from build123d import *

# Parameters (mm, degrees)
SKETCH_1_W          = 45
SKETCH_1_H          = 40
EXTRUDE_1_DEPTH     = 2
EXTRUDE_2_DEPTH     = 20
SKETCH_3_W          = 31
SKETCH_3_H          = 63
EXTRUDE_3_DEPTH     = 2
SKETCH_4_R          = 1.65
CUT_EXTRUDE_1_DEPTH = 2
FILLET_2_R          = 2
EXTRUDE_4_DEPTH     = 20
CUT_EXTRUDE_2_DEPTH = 2.5
CUT_EXTRUDE_5_REACH = 62.26
SKETCH_11_W         = 2
SKETCH_11_H         = 20
FILLET_5_R          = 1
CUT_EXTRUDE_6_DEPTH = 2.5


with BuildPart() as part:
    # 草图1 → 凸台-拉伸1 (new body)
    with BuildSketch(Plane(origin=(0, 0, 0), x_dir=(1, 0, 0), z_dir=(0, 1, 0))):
        Rectangle(SKETCH_1_W, SKETCH_1_H)
    extrude(amount=EXTRUDE_1_DEPTH)

    # 草图2 → 凸台-拉伸2 (add)
    with BuildSketch(Plane(origin=(0, 2, 0), x_dir=(1, 0, 0), z_dir=(0, 1, 0))):
        Polygon((21.5, -2.3), (22.5, -2.3), (22.5, 20), (-22.5, 20), (-22.5, -2.3), (-21.5, -2.3), (-21.5, 19), (21.5, 19), align=None)
    extrude(amount=EXTRUDE_2_DEPTH)

    # 草图3 → 凸台-拉伸3 (add)
    with BuildSketch(Plane.XZ):
        with Locations((0, 2)):
            Rectangle(SKETCH_3_W, SKETCH_3_H)
    extrude(amount=-EXTRUDE_3_DEPTH)

    # 草图4 → 切除-拉伸1 (cut)
    with BuildSketch(Plane.XZ):
        with Locations(Location((0, -23.15, 0), (0, 0, 270))):
            Circle(SKETCH_4_R)
        with Locations(Location((0, 24.35, 0), (0, 0, 90))):
            Circle(SKETCH_4_R)
    extrude(amount=-CUT_EXTRUDE_1_DEPTH, mode=Mode.SUBTRACT)

    # 圆角2
    fillet_2_edges = [part.edges().sort_by_distance(p)[0] for p in [
        (-15.5, 1, -29.5),
        (15.5, 1, 33.5),
        (-15.5, 1, 33.5),
        (15.5, 1, -29.5),
        (22.5, 1, 20),
        (-22.5, 1, 20),
        (-22.5, 11, -20),
        (22.5, 11, -20),
    ]]
    fillet(fillet_2_edges, radius=FILLET_2_R)

    # 草图7 → 凸台-拉伸4 (add)
    with BuildSketch(Plane(origin=(0, 2, 0), x_dir=(1, 0, 0), z_dir=(0, 1, 0))):
        Polygon((20.5, 18), (20.5, -2.3), (21.5, -2.3), (21.5, 19), (20.5, 19), align=None)
        Polygon((-21.5, 19), (-21.5, -2.3), (-20.5, -2.3), (-20.5, 18), (-20.5, 19), align=None)
    extrude(amount=EXTRUDE_4_DEPTH)

    # 草图8 → 切除-拉伸2 (cut)
    with BuildSketch(Plane(origin=(20, 1.9, 0.9), x_dir=(0, 1, 0), z_dir=(1, 0, 0))):
        with BuildLine():
            ThreePointArc((18.33276934, -17.5), (17.54276934, -16.71), (16.75276934, -17.5))
            ThreePointArc((16.75276934, -17.5), (17.54276934, -18.29), (18.33276934, -17.5))
        make_face()
        with BuildLine():
            ThreePointArc((3.33276934, -17.5), (2.54276934, -16.71), (1.75276934, -17.5))
            ThreePointArc((1.75276934, -17.5), (2.54276934, -18.29), (3.33276934, -17.5))
        make_face()
        with BuildLine():
            ThreePointArc((3.33276934, -2.5), (2.54276934, -1.71), (1.75276934, -2.5))
            ThreePointArc((1.75276934, -2.5), (2.54276934, -3.29), (3.33276934, -2.5))
        make_face()
        with BuildLine():
            ThreePointArc((18.33276934, -2.5), (17.54276934, -1.71), (16.75276934, -2.5))
            ThreePointArc((16.75276934, -2.5), (17.54276934, -3.29), (18.33276934, -2.5))
        make_face()
    extrude(amount=CUT_EXTRUDE_2_DEPTH, mode=Mode.SUBTRACT)

    # 切除-拉伸5: up to this face of the body (flat: up to its plane)
    cut_extrude_5_end = Plane(part.part.faces().sort_by_distance((22.5, 10.316412164, -6.626998027))[0])
    # 草图11 → 切除-拉伸5 (cut, up to the picked face)
    with BuildSketch(Plane.ZY.offset(22.5), mode=Mode.PRIVATE) as cut_extrude_5_sk1:
        with Locations((1.3, 12)):
            Rectangle(SKETCH_11_W, SKETCH_11_H)
    cut_extrude_5_tool1 = split(extrude(cut_extrude_5_sk1.sketch, amount=-CUT_EXTRUDE_5_REACH, mode=Mode.PRIVATE), bisect_by=cut_extrude_5_end, keep=Keep.BOTH, mode=Mode.PRIVATE)
    add(cut_extrude_5_tool1.solids().sort_by(Axis((-22.5, 12, 1.3), (1, 0, 0)))[0], mode=Mode.SUBTRACT)

    # 圆角5
    fillet_5_edges = [part.edges().sort_by_distance(p)[0] for p in [
        (20.5, 12, -19),
        (-20.5, 12, -19),
    ]]
    fillet(fillet_5_edges, radius=FILLET_5_R)

    # 草图12 → 切除-拉伸6 (cut)
    with BuildSketch(Plane(origin=(-20, 1.9, 0.9), x_dir=(0, -1, 0), z_dir=(-1, 0, 0))):
        with BuildLine():
            Line((-10.8, -17.95), (-10.8, -16.45))
            ThreePointArc((-10.8, -16.45), (-10, -15.65), (-9.2, -16.45))
            Line((-9.2, -16.45), (-9.2, -17.95))
            ThreePointArc((-9.2, -17.95), (-10, -18.75), (-10.8, -17.95))
        make_face()
        with BuildLine():
            Line((-3.8, -11.0010906), (-3.8, -10.0010906))
            ThreePointArc((-3.8, -10.0010906), (-3, -9.2010906), (-2.2, -10.0010906))
            Line((-2.2, -10.0010906), (-2.2, -11.0010906))
            ThreePointArc((-2.2, -11.0010906), (-3, -11.8010906), (-3.8, -11.0010906))
        make_face()
        with BuildLine():
            Line((-17.8, -11.0010906), (-17.8, -10.0010906))
            ThreePointArc((-17.8, -10.0010906), (-17, -9.2010906), (-16.2, -10.0010906))
            Line((-16.2, -10.0010906), (-16.2, -11.0010906))
            ThreePointArc((-16.2, -11.0010906), (-17, -11.8010906), (-17.8, -11.0010906))
        make_face()
    extrude(amount=CUT_EXTRUDE_6_DEPTH, mode=Mode.SUBTRACT)


solid = part.part
The model under review builds one solid part; all positions refer to its coordinate system, in mm. A direction names the side the tool comes from. Coordinates: 2 decimals unless noted, no trailing zeros. Write each loop counter-clockwise with the first axis right and the second up, starting at its lowest first coordinate (ties: lowest second). Pieces come first, ordered by that corner, then holes. Notation, with made-up numbers: (-30, -32.75) - (20, -32.75) arc R31 ccw to (20, 3.25) - close; hole circle Ø5 at (87.5, -11). An arc over 180 degrees is marked (long way). Answer as a JSON object with one key per item and string values. Group by question number.
1. Mouldability with a two-part tool opening along X and no side actions: class faces 1 (the face through (-21.9, 11.15, -19.43)), 2 (the face through (0, 2, 7)), 3 (the face through (-20.5, 12, -9)), 4 (the face through (-18, 1, 20)) as pulls with the +X half, pulls with the -X half, needs draft (parallel to the pull), parting line crosses it, or undercut.
2. Add section C-C (z = -1.6). Give the boundary of the cut face in (x, y).
3. To check wall thickness, follow probe 1 along X at (y, z) = (1.3, 24.35); probe 2 along Z at (x, y) = (-13.5, 20.5); probe 3 along X at (y, z) = (16.25, -12.5). State the ranges of each line that lie inside material, in increasing order.
4. Clearance check with flat-ended pins moving along their axes: pin 1 Ø22.5 at (x, z) = (-4, 15.5) entering from +Y; pin 2 Ø8 at (y, z) = (8, 8.5) entering from -X; pin 3 Ø8 at (x, z) = (1.5, -21.5) entering from -Y; pin 4 Ø6 at (x, y) = (-5, 9.5) entering from -Z. State where each tip first meets the part, or that it passes through.
5. Machinability: for faces 5 (the face through (18, 1, 20)), 6 (the face through (-21, 11.1, -16)), 7 (the face through (-22, 12, 0.3)), which of the approach directions +Z, -Z, +X, -X, +Y, -Y give a long, thin tool a straight path to every point of the face, cutting with its end or side? Answer none if there is none.
6. Add section B-B (z = -23.15). Give the boundary of the cut face in (x, y), plus the area to 3 significant figures.
7. Add section D-D (y = 12). Give the boundary of the cut face in (x, z), plus the area to 3 significant figures.
8. Add section A-A (x = 0). Give the boundary of the cut face in (y, z), plus the area to 3 significant figures.
Findings:
{
 "1": {"face 1": "pulls with the -X half", "face 2": "undercut", "face 3": "undercut", "face 4": "needs draft"},
 "2": {"outline": "(-22.5, 0) - (22.5, 0) - (22.5, 3.65) - (20.5, 3.65) - (20.5, 2) - (-20.5, 2) - (-20.5, 22) - (-22.5, 22) - close; (20.5, 5.23) - (22.5, 5.23) - (22.5, 18.65) - (20.5, 18.65) - close; (20.5, 20.23) - (22.5, 20.23) - (22.5, 22) - (20.5, 22) - close"},
 "3": {"probe 1": "-15.5 to -1.65, 1.65 to 15.5", "probe 2": "-20 to -19", "probe 3": "-22.5 to -20.5, 20.5 to 22.5"},
 "4": {"pin 1": "y = 2", "pin 2": "through", "pin 3": "y = 0", "pin 4": "z = -20"},
 "5": {"face 5": "+Z, +X, +Y, -Y", "face 6": "-X", "face 7": "+Z, +X, -X, +Y"},
 "6": {"outline": "(-15.5, 0) - (-1.65, 0) - (-1.65, 2) - (-15.5, 2) - close; (1.65, 0) - (15.5, 0) - (15.5, 2) - (1.65, 2) - close", "area": "55.4 mm²"},
 "7": {"outline": "(-22.5, -18) arc R2 ccw to (-20.5, -20) - (20.5, -20) arc R2 ccw to (22.5, -18) - (22.5, 0.3) - (20.5, 0.3) - (20.5, -18) arc R1 cw to (19.5, -19) - (-19.5, -19) arc R1 cw to (-20.5, -18) - (-20.5, -17.84) - (-22.5, -17.84) - close; (-22.5, -14.76) - (-20.5, -14.76) - (-20.5, 0.3) - (-22.5, 0.3) - close", "area": "115 mm²"},
 "8": {"outline": "(0, -29.5) - (2, -29.5) - (2, -24.8) - (0, -24.8) - close; (0, -21.5) - (2, -21.5) - (2, -20) - (22, -20) - (22, -19) - (2, -19) - (2, 22.7) - (0, 22.7) - close; (0, 26) - (2, 26) - (2, 33.5) - (0, 33.5) - close", "area": "133 mm²"}
}
